For this review, use the dimensioned drawing (mm, ordinates from the lowest corner) and the shaded views. A direction names the side the tool comes from. Coordinates: 2 decimals unless noted, no trailing zeros. Loops run counter-clockwise (first coordinate to the right, second up) from the corner with the lowest first, then second, coordinate; pieces in that order, holes last. Notation, with made-up numbers: M 11.25,27 L 52.25,27 A20 cw 52.25,47 Z; hole C -27,-33.75 d7. An arc over 180 degrees is marked long. Write item = value, one per line. Start each with the question number.
Q1. We need section D-D on y = 35.5. Give the boundary of the cut face in (x, z) (3 decimals), and give its area (3 significant figures).
Q2. Clearance check with flat-ended pins moving along their axes: pin 1 Ø4.5 at (x, z) = (43.5, 3) entering from -Y; pin 2 Ø3 at (y, z) = (23, 2.5) entering from -X; pin 3 Ø2 at (x, y) = (19, 33) entering from +Z. State where each tip first meets the part, or that it passes through.
Q3. We need section A-A on y = 20. Give the boundary of the cut face in (x, z) (3 decimals), and give its area (3 significant figures).
Q4. We need section C-C on z = 4.75. Give the boundary of the cut face in (x, y) (3 decimals), and give its area (3 significant figures).
Q5. Mouldability with a two-part tool opening along X and no side actions: class the marked faces 1, 2 and 3 as released by +X, released by -X, zero draft, split by the parting line, or undercut.
Q6. For the marked faces 4, 5, 6 and 7, list the 3-axis set-ups (+Z, -Z, +X, -X, +Y, -Y) from which the entire face can be reached by the end or side of a thin tool; tool diameter is ignored.
Q7. We need section B-B on x = 20. Give the boundary of the cut face in (y, z), and give its area (3 significant figures).
Q8. Wall thickness on probe 1 along Y at (x, z) = (20, 2.1); probe 2 along Y at (x, z) = (41, 0.75); probe 3 along X at (y, z) = (9, 4) (1 decimal): over which ranges is each line inside the solid? List them lowest first.
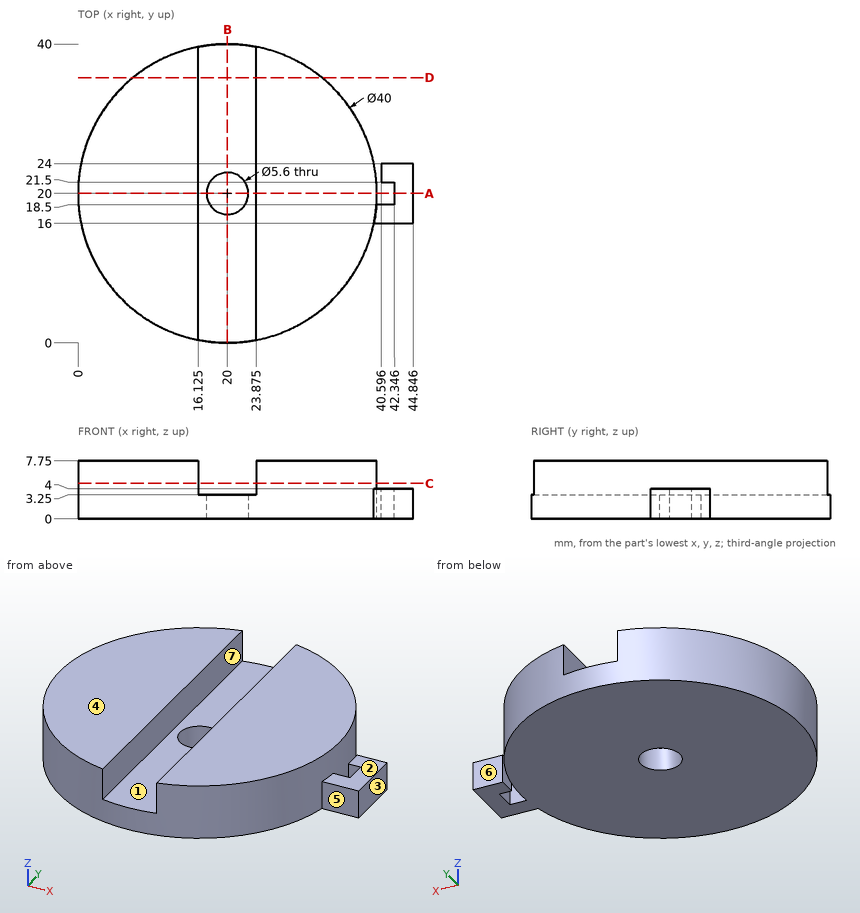
Returned:
q1.outline = M 7.361,0 L 32.639,0 L 32.639,7.75 L 23.875,7.75 L 23.875,3.25 L 16.125,3.25 L 16.125,7.75 L 7.361,7.75 Z
q1.area = 161 mm^2
q2.pin_1 = 16
q2.pin_2 = 0.06
q2.pin_3 = 3.25
q3.outline = M 0,0 L 17.2,0 L 17.2,3.25 L 16.125,3.25 L 16.125,7.75 L 0,7.75 Z; M 22.8,0 L 40,0 L 40,7.75 L 23.875,7.75 L 23.875,3.25 L 22.8,3.25 Z; M 42.346,0 L 44.846,0 L 44.846,4 L 42.346,4 Z
q3.area = 267 mm^2
q4.outline = M 16.125,0.379 L 16.125,39.621 A20 ccw Z; M 23.875,0.379 A20 ccw 23.875,39.621 Z
q4.area = 949 mm^2
q5.face_1 = undercut
q5.face_2 = zero draft
q5.face_3 = released by +X
q6.face_4 = +Z, +X, -X, +Y, -Y
q6.face_5 = +Z, -Z, +X, -Y
q6.face_6 = +Z, -Z, +X, +Y
q6.face_7 = +Z, +Y, -Y
q7.outline = M 0,0 L 17.2,0 L 17.2,3.25 L 0,3.25 Z; M 22.8,0 L 40,0 L 40,3.25 L 22.8,3.25 Z
q7.area = 112 mm^2
q8.probe_1 = 0 to 17.2, 22.8 to 40
q8.probe_2 = 16 to 18.5, 21.5 to 24
q8.probe_3 = 3.3 to 16.1, 23.9 to 36.7
